CAD build for the part. Positions are in the model's coordinates, mm. Face numbers are marked on the shaded views. A direction names the side the tool comes from. Round coordinates to 2 decimals unless told otherwise and drop trailing zeros. Loops run counter-clockwise (first coordinate to the right, second up) from the corner with the lowest first, then second, coordinate; pieces in that order, holes last. Notation, with made-up numbers: (0.5, 14) - (30.5, 14) arc R13 ccw to (30.5, 34) - close; hole circle Ø9 at (-13, 54.5). An arc over 180 degrees is marked (long way). Use one line per item in the form item = value.
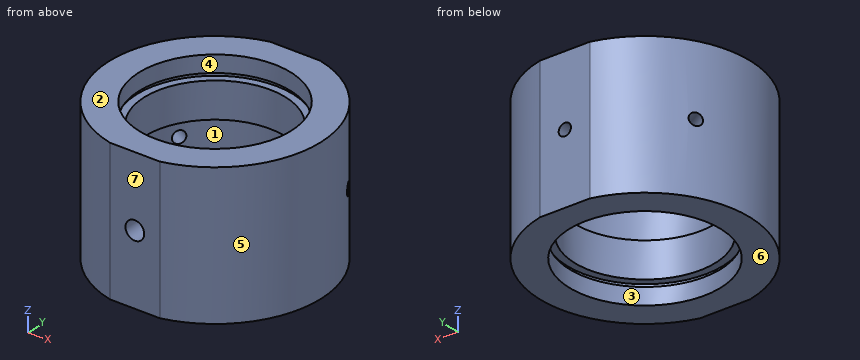
from build123d import *

# Parameters (mm, degrees)
SKETCH_2_W                       = 64.02174429
SKETCH_2_H                       = 9.248919907
CUT_EXTRUDE_1_DEPTH              = 49
HOLE_WIZARD_M4_2_D               = 3.3
HOLE_WIZARD_M4_2_DEPTH           = 5.5
HOLE_WIZARD_M4_2_TIP             = 0.991420021
HOLE_WIZARD_M6_2_D               = 5
HOLE_WIZARD_M6_2_DEPTH           = 5.5
HOLE_WIZARD_M6_2_TIP             = 1.502151548
HOLE_WIZARD_M4_3_D               = 3.3
HOLE_WIZARD_M4_3_DEPTH           = 10.1
HOLE_WIZARD_M4_3_TIP             = 0.991420021
HOLE_WIZARD_M4_3_ON_FACE_2_D     = 3.3
HOLE_WIZARD_M4_3_ON_FACE_2_DEPTH = 10.1
HOLE_WIZARD_M4_3_ON_FACE_2_TIP   = 0.991420021


with BuildPart() as part:
    # 草图1 → 旋转1 (revolve)
    with BuildSketch(Plane(origin=(0, 0, 0), x_dir=(1, 0, 0), z_dir=(0, 1, 0)), mode=Mode.PRIVATE) as revolve_1_sk:
        Polygon((28.5, 19), (28.5, -19), (20.5, -19), (20.5, -14.5), (21.1, -14.5), (21.1, -13.5), (19.05, -13.5), (19.05, -4), (20.15, -4), (20.15, 4), (19.05, 4), (19.05, 13.5), (21.1, 13.5), (21.1, 14.5), (20.5, 14.5), (20.5, 19), align=None)
    revolve(revolve_1_sk.sketch.rotate(Axis((0, 0, -31.9390681), (0, 0, 1)), 180), axis=Axis((0, 0, -31.9390681), (0, 0, 1)))  # turned: the seam where the file's is

    # 草图2 → 切除-拉伸1 (cut)
    with BuildSketch(Plane.XY.offset(19)):
        with Locations((-1.141100508, 32.324459954)):
            Rectangle(SKETCH_2_W, SKETCH_2_H)
        with Locations((-1.141100508, -32.324459954)):
            Rectangle(SKETCH_2_W, SKETCH_2_H)
    extrude(amount=-CUT_EXTRUDE_1_DEPTH, mode=Mode.SUBTRACT)

    # M4 螺纹孔2
    with Locations(Plane(origin=(0, 27.7, 0), x_dir=(1, 0, 0), z_dir=(0, 1, 0))):
        with Locations((0, 0)):
            Hole(HOLE_WIZARD_M4_2_D / 2, depth=HOLE_WIZARD_M4_2_DEPTH)
            with Locations((0, 0, -(HOLE_WIZARD_M4_2_DEPTH + HOLE_WIZARD_M4_2_TIP / 2))):  # 118° drill point
                Cone(0, HOLE_WIZARD_M4_2_D / 2, HOLE_WIZARD_M4_2_TIP, mode=Mode.SUBTRACT)

    # M6 螺纹孔2
    with Locations(Plane(origin=(0, -27.7, 0), x_dir=(-1, 0, 0), z_dir=(0, -1, 0))):
        with Locations((0, 0)):
            Hole(HOLE_WIZARD_M6_2_D / 2, depth=HOLE_WIZARD_M6_2_DEPTH)
            with Locations((0, 0, -(HOLE_WIZARD_M6_2_DEPTH + HOLE_WIZARD_M6_2_TIP / 2))):  # 118° drill point
                Cone(0, HOLE_WIZARD_M6_2_D / 2, HOLE_WIZARD_M6_2_TIP, mode=Mode.SUBTRACT)

    # M4 螺纹孔3
    with Locations(Plane(origin=(24.681724008, 14.25, 0), x_dir=(-0.5, 0.866025404, 0), z_dir=(0.866025404, 0.5, 0))):
        with Locations((0, 0)):
            Hole(HOLE_WIZARD_M4_3_D / 2, depth=HOLE_WIZARD_M4_3_DEPTH)
            with Locations((0, 0, -(HOLE_WIZARD_M4_3_DEPTH + HOLE_WIZARD_M4_3_TIP / 2))):  # 118° drill point
                Cone(0, HOLE_WIZARD_M4_3_D / 2, HOLE_WIZARD_M4_3_TIP, mode=Mode.SUBTRACT)

    # M4 螺纹孔3 on face 2
    with Locations(Plane(origin=(-24.681724008, 14.25, 0), x_dir=(-0.500000175, -0.866025303, 0), z_dir=(-0.866025303, 0.500000175, 0))):
        with Locations((0, 0)):
            Hole(HOLE_WIZARD_M4_3_ON_FACE_2_D / 2, depth=HOLE_WIZARD_M4_3_ON_FACE_2_DEPTH)
            with Locations((0, 0, -(HOLE_WIZARD_M4_3_ON_FACE_2_DEPTH + HOLE_WIZARD_M4_3_ON_FACE_2_TIP / 2))):  # 118° drill point
                Cone(0, HOLE_WIZARD_M4_3_ON_FACE_2_D / 2, HOLE_WIZARD_M4_3_ON_FACE_2_TIP, mode=Mode.SUBTRACT)


solid = part.part
1) Slice it at B-B (z = 9). Write the cut outline in (x, y), plus the area to 3 significant figures.
Report:
outline = (-6.71, -27.7) - (6.71, -27.7) arc R28.5 ccw to (6.71, 27.7) - (-6.71, 27.7) arc R28.5 ccw to start; hole circle Ø38.1 at (0, 0)
area = 1,400 mm^2
2) Drill centre lines: probe 1 along Z at (x, y) = (16, 13); probe 2 along Y at (x, z) = (0, -17.45); probe 3 along Y at (x, z) = (0, -13.85). Where is each one in solid material? Low to high.
Report:
probe_1 = -19 to -14.5, -13.5 to 13.5, 14.5 to 19
probe_2 = -27.7 to -20.5, 20.5 to 27.7
probe_3 = -27.7 to -21.1, 21.1 to 27.7
3) Tool access for the marked faces 1, 2 and 3: list every direction of +Z, -Z, +X, -X, +Y, -Y with a clear straight run to the whole face (end or side of a thin tool).
Report:
face_1 = none
face_2 = +Z, +X, -X, +Y, -Y
face_3 = -Z
4) Flat gauge pins, fed straight in: pin 1 (21 mm diameter, centred on x = 4, y = -4.5, fed in from -Z); pin 2 (10 mm diameter, centred on y = 5, z = 2.5, fed in from -X); pin 3 (2 mm diameter, centred on y = 13, z = 7.5, fed in from +X); pin 4 (10 mm diameter, centred on y = -7.5, z = 12, fed in from -X). Where does each tip first touch, or does it go through?
Report:
pin_1 = through
pin_2 = -28.5
pin_3 = 25.85
pin_4 = -28.39
5) Two-plate mould, pull along Y, no slides. Class the marked faces 4, 5, 6 and 7: +Y half, -Y half, draft (parallel to the pull), parting line (faces both ways), or undercut.
Report:
face_4 = undercut
face_5 = parting line
face_6 = draft
face_7 = -Y half
6) Slice it at D-D (z = 16). Write the cut outline in (x, y), plus the area to 3 significant figures.
Report:
outline = (-6.71, -27.7) - (6.71, -27.7) arc R28.5 ccw to (6.71, 27.7) - (-6.71, 27.7) arc R28.5 ccw to start; hole circle Ø41 at (0, 0)
area = 1,220 mm^2
